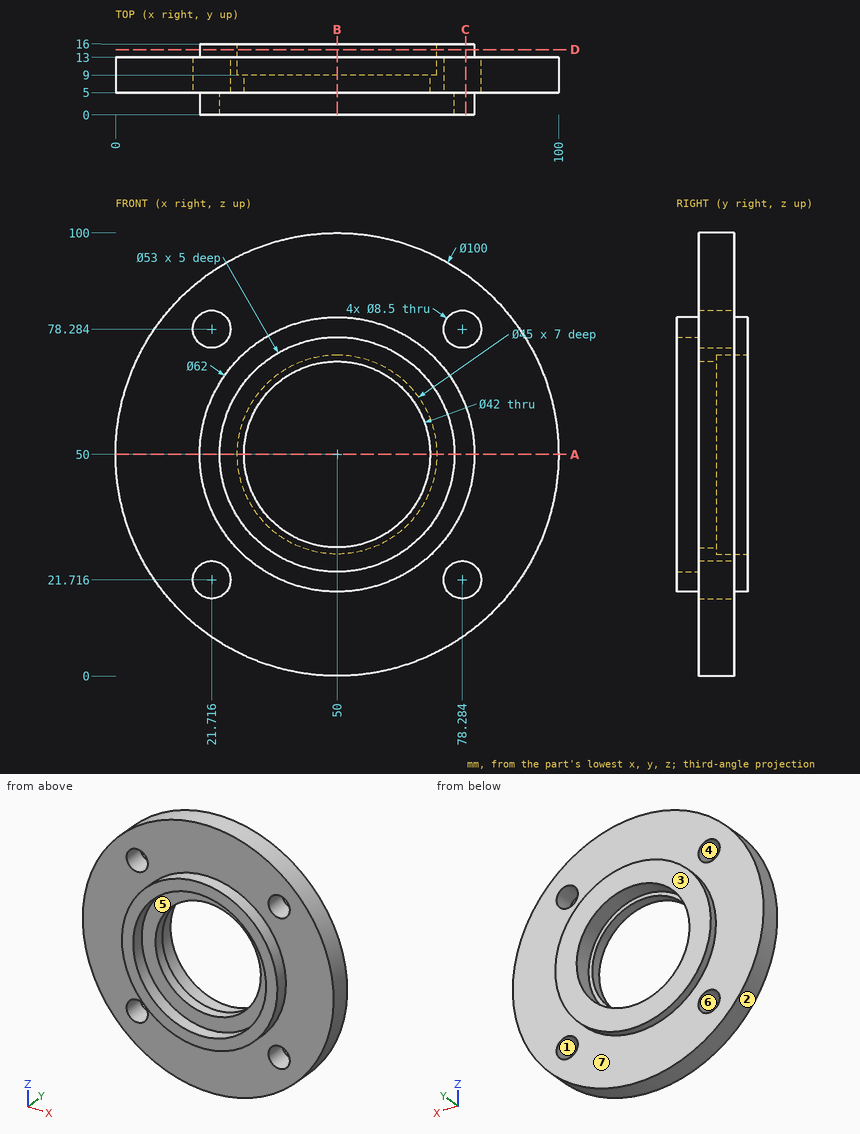
Study the drawing (mm; zero at the part's minimum x, y, z) and answer. A direction names the side the tool comes from. Round coordinates to 2 decimals unless told otherwise and drop trailing zeros. Order: outer loops, then holes, each group sorted by start corner. A loop starts at its lowest first (then second) coordinate and runs counter-clockwise, first axis right, second up. Notation, with made-up numbers: (10.5, 75.5) - (34.5, 75.5) arc R20 cw to (34.5, 95.5) - close; hole circle Ø3 at (12.5, -16). An arc over 180 degrees is marked (long way). Use one line per item in the form item = value. Start each with the question number.
(1) The part is cut by section A-A (z = 50). Give the vertices of the cut face in (x, y), then the cut area to 3 significant figures.
(2) The part is cut by section B-B (x = 50). Give the vertices of the cut face in (y, z), then the cut area to 3 significant figures.
(3) For the marked faces 5, 6 and 7, determine the directions among +Z, -Z, +X, -X, +Y, -Y from which every point of the face is accessible in a straight line to the end or side of a thin tool.
(4) Find the intervals of material crossed by line 1 along X through (y, z) = (6, 77.5); line 2 along Z through (x, y) = (24, 9.25); line 3 along Z through (x, y) = (75.5, 11.5) (1 decimal), in increasing order. Write a range as from..to.
(5) The part is cut by section C-C (x = 79). Give the vertices of the cut face in (y, z) (1 decimal), then the cut area to 3 significant figures.
(6) Determine the mould class of the marked faces 1, 2, 3 and 4 for opening direction X: +X half, -X half, draft (parallel to the pull), parting line (faces both ways), or undercut.
(7) Flat-ended cylindrical pins translate along their axes: pin 1 Ø6 at (y, z) = (7, 66) entering from +X; pin 2 Ø7.5 at (x, z) = (21.72, 21.72) entering from +Y; pin 3 Ø10 at (x, z) = (84, 15.5) entering from +Y; pin 4 Ø6 at (y, z) = (11.5, 79) entering from -X. Find the tip coordinate at first contact, or state that the pin passes through.
(8) The part is cut by section D-D (y = 14.75). Give the vertices of the cut face in (x, z).
Checked values:
q1.outline = (0, 5) - (19, 5) - (19, 0) - (23.5, 0) - (23.5, 5) - (29, 5) - (29, 9) - (27.5, 9) - (27.5, 16) - (19, 16) - (19, 13) - (0, 13) - close; (71, 5) - (76.5, 5) - (76.5, 0) - (81, 0) - (81, 5) - (100, 5) - (100, 13) - (81, 13) - (81, 16) - (72.5, 16) - (72.5, 9) - (71, 9) - close
q1.area = 548 mm^2
q2.outline = (0, 19) - (5, 19) - (5, 0) - (13, 0) - (13, 19) - (16, 19) - (16, 27.5) - (9, 27.5) - (9, 29) - (5, 29) - (5, 23.5) - (0, 23.5) - close; (0, 76.5) - (5, 76.5) - (5, 71) - (9, 71) - (9, 72.5) - (16, 72.5) - (16, 81) - (13, 81) - (13, 100) - (5, 100) - (5, 81) - (0, 81) - close
q2.area = 548 mm^2
q3.face_5 = -Y
q3.face_6 = +Y, -Y
q3.face_7 = +Y
q4.line_1 = 8.24..17.54, 25.89..74.11, 82.46..91.76
q4.line_2 = 7.29..18.13, 25.3..74.7, 81.87..92.71
q4.line_3 = 7..18.5, 24.9..75.1, 81.5..93
q5.outline = (0, 39) - (5, 39) - (5, 25.9) - (13, 25.9) - (13, 39) - (16, 39) - (16, 61) - (13, 61) - (13, 74.1) - (5, 74.1) - (5, 61) - (0, 61) - close; (5, 9.3) - (13, 9.3) - (13, 17.5) - (5, 17.5) - close; (5, 82.5) - (13, 82.5) - (13, 90.7) - (5, 90.7) - close
q5.area = 693 mm^2
q6.face_1 = undercut
q6.face_2 = parting line
q6.face_3 = draft
q6.face_4 = undercut
q7.pin_1 = 98.28
q7.pin_2 = through
q7.pin_3 = 13
q7.pin_4 = 7.29
q8.outline = circle Ø62 at (50, 50); hole circle Ø45 at (50, 50)
